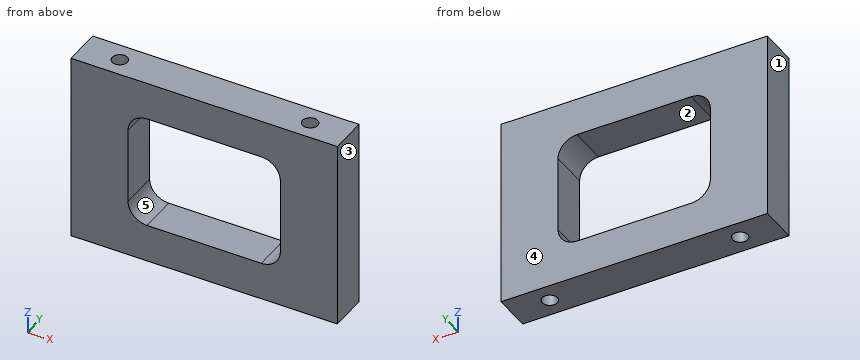
Autodesk Fusion 360 part; units mm, degrees
sketch "Sketch1" plane through (0, 0, 0) normal (0, 0, 1) x (1, 0, 0)
  line L0 (0, 0) -> (70, 0)
  line L1 (70, 0) -> (70, 10)
  line L2 (70, 10) -> (0, 10)
  line L3 (0, 10) -> (0, 0)
  line L4 (0, 5) -> (70, 5) construction
  point P0 (10, 5)
  point P1 (60, 5)
  dimension "d1" = 70
  dimension "d2" = 10
  dimension "d9" = 50
  dimension "d10" = 10
extrude "Extrude1" add sketch "Sketch1" along normal blind 50
sketch "Sketch2" plane through (0, 0, 50) normal (0, 0, 1) x (-1, 0, 0)
  line L0 (0, -10) -> (0, 0)
  line L1 (0, 0) -> (-70, 0)
  line L2 (-70, 0) -> (-70, -10)
  line L3 (-70, -10) -> (0, -10)
  line L4 (0, -5) -> (-70, -5) construction
  line L5 (0, -10) -> (0, 0)
  point P0 (-10, -5)
  point P1 (-60, -5)
  dimension "d11" = 50
  dimension "d12" = 10
hole "Hole1" at (10, 5, 50) at (60, 5, 50) direction (0, 0, -1) diameter 4 depth 6 tip angle 180
hole "Hole2" at (10, 5, 0) at (60, 5, 0) direction (0, 0, 1) diameter 4 depth 6 tip angle 180
sketch "Sketch3" plane through (0, 0, 0) normal (0, -1, 0) x (1, 0, 0)
  line L0 (0, 0) -> (70, 0)
  line L1 (70, 0) -> (70, 50)
  line L2 (70, 50) -> (0, 50)
  line L3 (0, 50) -> (0, 0)
  line L4 (15, 40) -> (55, 40)
  line L5 (55, 40) -> (55, 10)
  line L6 (55, 10) -> (15, 10)
  line L7 (15, 10) -> (15, 40)
  line L8 (0, 0) -> (70, 0)
  dimension "d19" = 15
  dimension "d20" = 10
  dimension "d21" = 10
  dimension "d22" = 15
extrude "Extrude2" cut sketch "Sketch3" against normal blind 33 contours L4 L5 L6 L7
fillet "Fillet1" radius 5 4 edges at (15, 5, 40) (55, 5, 40) (55, 5, 10) (15, 5, 10)
equation "d10 = ( 70 mm - d9 ) / 2"
equation "d12 = ( 70 mm - d11 ) / 2"
Build history of the part. All positions in model axes, mm. Face numbers are marked on the shaded views. A direction names the side the tool comes from. Round coordinates to 2 decimals unless told otherwise and drop trailing zeros. Write each loop counter-clockwise with the first axis right and the second up, starting at its lowest first coordinate (ties: lowest second). Pieces come first, ordered by that corner, then holes. Notation, with made-up numbers: (56.25, 42) - (74.25, 42) arc R22 cw to (74.25, 60) - close; hole circle Ø1 at (43.5, 28). An arc over 180 degrees is marked (long way). Use CSV: the item, a comma, the result in double quotes.
(1) Band-saw the part on C-C (x = 26). Write the cut outline in (y, z), plus the area to 3 significant figures.
Response:
outline,"(0, 0) - (10, 0) - (10, 10) - (0, 10) - close; (0, 40) - (10, 40) - (10, 50) - (0, 50) - close"
area,"200 mm²"
(2) Pin check, flat tips, straight feed: P1, Ø1.2, axis at x = 11, y = 5, coming from the -Z side; P2, Ø2.5, axis at x = 60, y = 5, coming from the +Z side; P3, Ø3, axis at x = 38, y = 6.5, coming from the -Z side. Stop position of each tip, or through.
Response:
P1,"z = 6"
P2,"z = 44"
P3,"z = 0"
(3) Band-saw the part on A-A (z = 28.5). Write the cut outline in (x, y), plus the area to 3 significant figures.
Response:
outline,"(0, 0) - (15, 0) - (15, 10) - (0, 10) - close; (55, 0) - (70, 0) - (70, 10) - (55, 10) - close"
area,"300 mm²"
(4) 3-axis set-ups, long thin cutter, end or side, ignore diameter. For the marked faces 1 and 2: which of +Z, -Z, +X, -X, +Y, -Y reach the whole face in a straight line?
Response:
face 1,"+Z, -Z, -X, +Y, -Y"
face 2,"+Y, -Y"
(5) Wall check: line 1 (X direction, y = 5, z = 47.8); line 2 (Y direction, x = 10, z = 47.15); line 3 (X direction, y = 9, z = 30). Give the ranges that are in metal, low to high.
Response:
line 1,"0 to 8, 12 to 58, 62 to 70"
line 2,"0 to 3, 7 to 10"
line 3,"0 to 15, 55 to 70"
(6) Band-saw the part on B-B (y = 1). Write the cut outline in (x, z).
Response:
outline,"(0, 0) - (70, 0) - (70, 50) - (0, 50) - close; hole (15, 15) arc R5 ccw to (20, 10) - (50, 10) arc R5 ccw to (55, 15) - (55, 35) arc R5 ccw to (50, 40) - (20, 40) arc R5 ccw to (15, 35) - close"
(7) Band-saw the part on D-D (z = 4). Write the cut outline in (x, y).
Response:
outline,"(0, 0) - (70, 0) - (70, 10) - (0, 10) - close; hole circle Ø4 at (10, 5); hole circle Ø4 at (60, 5)"
(8) Mould opens along X. For the marked faces 3, 4 and 5 say: pulls with the +X half, pulls with the -X half, needs draft (parallel to the pull), parting line crosses it, or undercut.
Response:
face 3,"pulls with the +X half"
face 4,"needs draft"
face 5,"undercut"
